Verification items for the finished model (mm, model axes). A direction names the side the tool comes from. Coordinates: 2 decimals unless noted, no trailing zeros. Order: outer loops, then holes, each group sorted by start corner. A loop starts at its lowest first (then second) coordinate and runs counter-clockwise, first axis right, second up. Notation, with made-up numbers: M 19.25,2 L 66.25,2 A21 cw 66.25,11 Z; hole C -35,53 d4. An arc over 180 degrees is marked long. Return JSON: item names as keys, results as strings. Group by question number.
Q1. Mould release check, pull along X, two halves, no side actions. Record for faces 1 (the face through (1.4, -31.4, -3)), 2 (the face through (-24.6, 13.6, -3)), 3 (the face through (25, 0, 0)): pulls with the +X half, pulls with the -X half, needs draft (parallel to the pull), parting line crosses it, or undercut.
Q2. Access from +Z, -Z, +X, -X, +Y, -Y to the whole of each face (thin tool, end or side, straight path). Record for faces 4 (the face through (1.245, -33.002, -1.521)), 5 (the face through (23, 8, -2)), 6 (the face through (1.055, -23.977, -1.014)).
Q3. Thickness scan on probe 1 along X at (y, z) = (-15, -5.75); probe 2 along Y at (x, z) = (-3, -1); probe 3 along X at (y, z) = (-15, -1.3) (3 decimals). Record the ranges inside material, lowest first.
Q4. Go/stop test with flat-tipped pins: pin 1 Ø5.5 at (x, y) = (25.98, -15) entering from +Z; pin 2 Ø3 at (x, z) = (6.5, -3) entering from -Y; pin 3 Ø1.5 at (y, z) = (-18.5, -13) entering from -X. Record where each tip stops, or that it passes through.
Q5. Section check B-B, the plane z = -7. Enter the section's corners in (x, y), then the cut area to 3 significant figures.
Q6. Section check A-A, the plane x = 0. Count the separate pieces of the cut face and the enclosed holes in it, then the cut area to 3 significant figures.
Autodesk Inventor part; units mm, degrees
ref_plane "YZ Plane" through (0, 0, 0) normal (1, 0, 0) x (0, 1, 0)
ref_plane "XZ Plane" through (0, 0, 0) normal (0, 1, 0) x (-1, 0, 0)
ref_plane "XY Plane" through (0, 0, 0) normal (0, 0, 1) x (1, 0, 0)
sketch "スケッチ2" plane through (0, 0, 0) normal (1, 0, 0) x (0, 1, 0)
  line L0 (0, 0) -> (26, 0)
  line L1 (26, 0) -> (26, -16)
  line L2 (26, -16) -> (0, -16)
  line L3 (0, -16) -> (0, 0)
  line L4 (0, 0) -> (34, 0)
  line L5 (34, 0) -> (34, -16)
  line L6 (34, -16) -> (0, -16)
  line L7 (0, -16) -> (0, 0)
  line L8 (34, 0) -> (21, 0)
  line L9 (26, 0) -> (24, 0)
  line L10 (24, 0) -> (24, -2)
  line L11 (24, -2) -> (26, -2)
  line L12 (26, -2) -> (26, 0)
  point P0 (26, 0)
  point P1 (26, -16)
  point P2 (26, -2)
  point P3 (24, 0)
  dimension "d1" = 26
  dimension "d8" = 2
  dimension "d10" = 14
  dimension "d27" = 8
  dimension "d31" = 2
revolve "回転1" add sketch "スケッチ2" angle 360 about axis through (0, 0, -16) along (0, 0, 1) contours L0 L1 L11 L10 | L1 L4 L5 L6
sketch "スケッチ4" plane through (0, 0, 0) normal (0, 0, 1) x (1, 0, 0)
  point P0 (0, 0)
  point P1 (0, 30)
  point P2 (-25.9808, 15)
  point P3 (-25.9808, -15)
  point P4 (0, -30)
  point P5 (25.9808, -15)
  point P6 (25.9808, 15)
  dimension "d11" = 30
  dimension "d14" = 360
hole "穴1" at (0, 30, 0) at (-25.9808, 15, 0) at (-25.9808, -15, 0) at (0, -30, 0) at (25.9808, -15, 0) at (25.9808, 15, 0) direction (0, 0, -1) diameter 3.4 end through all counterbore diameter 6.5 counterbore depth 3
chamfer "面取り1" distance 0.5 angle 45 1 edges at (0, -26, -16)
chamfer "面取り2" distance 0.5 angle 45 1 edges at (0, -34, 0)
properties part number "bearing_cover_j5" material "ABS プラスチック"
Numbers:
{
 "1": {"face 1": "undercut", "face 2": "undercut", "face 3": "needs draft"},
 "2": {"face 4": "+Z", "face 5": "-Z", "face 6": "+Z, -Z"},
 "3": {"probe 1": "x = -30.51 to -27.68, -24.28 to -21.24, 21.24 to 24.28, 27.68 to 30.51", "probe 2": "y = -33.87 to -31.25, -28.75 to -23.81, 23.81 to 28.75, 31.25 to 33.87", "probe 3": "x = -30.512 to -29.231, -22.731 to -18.735, 18.735 to 22.731, 29.231 to 30.512"},
 "4": {"pin 1": "stops at z = -3", "pin 2": "stops at y = -33.63", "pin 3": "stops at x = -29"},
 "5": {"outline": "C 0,0 d68; hole C -25.98,-15 d3.4; hole C -25.98,15 d3.4; hole C 0,0 d52; hole C 0,-30 d3.4; hole C 0,30 d3.4; hole C 25.98,-15 d3.4; hole C 25.98,15 d3.4", "area": "1,450 mm2"},
 "6": {"separate pieces": "4", "enclosed holes": "0", "area": "136 mm2"}
}
